Autodesk Fusion 360 part; units mm, degrees
sketch "Sketch1" plane through (0, 0, 0) normal (0, 1, 0) x (1, 0, 0)
sketch "Sketch2" plane through (0, 0, 0) normal (0, 1, 0) x (1, 0, 0)
sketch "Sketch3" plane through (0, 0, 0) normal (0, 1, 0) x (1, 0, 0)
  line L0 (-7.8, -52.8) -> (7.8, -52.8)
  line L1 (7.8, -52.8) -> (7.8, -37.2)
  line L2 (7.8, -37.2) -> (-7.8, -37.2)
  line L3 (-7.8, -37.2) -> (-7.8, -52.8)
  line L4 (-7.8, -52.8) -> (7.8, -37.2) construction
  line L5 (7.8, -52.8) -> (-7.8, -37.2) construction
  point P0 (0, -45)
  dimension "d3" = 15.6
  dimension "d4" = 15.6
extrude "Extrude1" add sketch "Sketch3" along normal blind 6.6 draft -20 makes body 1
sketch "Sketch4" plane through (0, 0, 0) normal (1, 0, 0) x (0, 0, -1)
extrude "Extrude2" add 1 faces at (-2.6, 0, 42.4) along direction (0, -1, 0) blind 5 draft -10 on bodies 1 bodies 1
sketch "Sketch5" plane through (0, 6.6, 0) normal (0, 1, 0) x (-1, 0, 0)
  line L0 (-5.3978, 39.6022) -> (5.3978, 39.6022)
  line L1 (5.3978, 39.6022) -> (5.3978, 50.3978)
  line L2 (5.3978, 50.3978) -> (-5.3978, 50.3978)
  line L3 (-5.3978, 50.3978) -> (-5.3978, 39.6022)
  line L4 (-3, 41) -> (3, 41)
  line L5 (3, 41) -> (3, 49)
  line L6 (3, 49) -> (-3, 49)
  line L7 (-3, 49) -> (-3, 41)
  line L8 (-3, 41) -> (3, 49) construction
  line L9 (3, 41) -> (-3, 49) construction
  point P0 (0, 45)
extrude "Extrude3" cut sketch "Sketch5" against normal blind 1 contours L4 L5 L6 L7 bodies 1
sketch "Sketch6" plane through (0, 5.6, 0) normal (0, 1, 0) x (-1, 0, 0)
  line L0 (-3, 49) -> (-3, 41)
  line L1 (-3, 41) -> (3, 41)
  line L2 (3, 41) -> (3, 49)
  line L3 (3, 49) -> (-3, 49)
  line L4 (2.8, 41.1) -> (-2.8305, 41.1)
  line L5 (-2.8305, 41.1) -> (-2.8305, 48.9)
  line L6 (-2.8305, 48.9) -> (2.8, 48.9)
  line L7 (2.8, 48.9) -> (2.8, 41.1)
  line L8 (2.8, 41.1) -> (-2.8305, 48.9) construction
  line L9 (-2.8305, 41.1) -> (2.8, 48.9) construction
  point P0 (-0.0152, 45)
extrude "Extrude4" add sketch "Sketch6" along normal blind 2 contours L4 L5 L6 L7 bodies 1
sketch "Sketch7" plane through (0, 7.6, 0) normal (0, 1, 0) x (-1, 0, 0)
  line L0 (2.8, 48.9) -> (-2.8305, 48.9)
  line L1 (-2.8305, 48.9) -> (-2.8305, 41.1)
  line L2 (-2.8305, 41.1) -> (2.8, 41.1)
  line L3 (2.8, 41.1) -> (2.8, 48.9)
  line L4 (0.6, 43.2) -> (-0.6, 43.2)
  line L5 (-0.6, 43.2) -> (-0.6, 46.8)
  line L6 (-0.6, 46.8) -> (0.6, 46.8)
  line L7 (0.6, 46.8) -> (0.6, 43.2)
  line L8 (0.6, 43.2) -> (-0.6, 46.8) construction
  line L9 (-0.6, 43.2) -> (0.6, 46.8) construction
  line L10 (-1.8, 44.4) -> (1.8, 44.4)
  line L11 (1.8, 44.4) -> (1.8, 45.6)
  line L12 (1.8, 45.6) -> (-1.8, 45.6)
  line L13 (-1.8, 45.6) -> (-1.8, 44.4)
  line L14 (-1.8, 44.4) -> (1.8, 45.6) construction
  line L15 (1.8, 44.4) -> (-1.8, 45.6) construction
  point P0 (0, 45)
  point P1 (0, 45)
extrude "Extrude5" add sketch "Sketch7" along normal blind 3.2 contours L4 L5 L7 L10 | L5 L7 L10 L12 | L7 L10 L11 L12 | L5 L10 L12 L13 | L5 L6 L7 L12 bodies 1
sketch "Sketch8" plane through (-2.8, 0, 0) normal (-1, 0, 0) x (0, 0, 1)
  line L0 (41.1, 5.6) -> (48.9, 5.6)
  line L1 (48.9, 5.6) -> (48.9, 7.6)
  line L2 (48.9, 7.6) -> (41.1, 7.6)
  line L3 (41.1, 7.6) -> (41.1, 5.6)
extrude "Extrude6" cut 1 faces at (1.4, 10.8, 45.2) along direction (0, -1, 0) blind 0.6 on bodies 1 bodies 1
sketch "Sketch9" plane through (0, -5, 0) normal (0, -1, 0) x (1, 0, 0)
  line L0 (6.9184, 51.9184) -> (-6.9184, 51.9184)
  line L1 (-6.9184, 51.9184) -> (-6.9184, 38.0816)
  line L2 (-6.9184, 38.0816) -> (6.9184, 38.0816)
  line L3 (6.9184, 38.0816) -> (6.9184, 51.9184)
  circle A0 centre (0, 45) radius 3
extrude "Extrude7" add sketch "Sketch9" along normal blind 2.5 contours A0 bodies 1
extrude "Extrude8" add 1 faces at (0.8808, -7.5, 44.8347) along direction (0, -1, 0) blind 0.8 draft -45 on bodies 1 bodies 1
sketch "Sketch10" plane through (0, -5, 0) normal (0, -1, 0) x (1, 0, 0)
  circle A0 centre (0, 45) radius 3
  line L0 (6.9184, 51.9184) -> (-6.9184, 51.9184)
  line L1 (-6.9184, 51.9184) -> (-6.9184, 38.0816)
  line L2 (-6.9184, 38.0816) -> (6.9184, 38.0816)
  line L3 (6.9184, 38.0816) -> (6.9184, 51.9184)
  circle A1 centre (-5, 42.5) radius 0.5
  circle A2 centre (5, 40) radius 0.5
extrude "Extrude9" add sketch "Sketch10" along normal blind 2.5 contours A1 | A2 bodies 1
extrude "Extrude10" add 2 faces at (-5.0609, -7.5, 42.6551) (4.9391, -7.5, 40.1551) along direction (0, -1, 0) blind 0.8 draft -25 on bodies 1 bodies 1
sketch "Sketch11" plane through (-2.8, 0, 0) normal (-1, 0, 0) x (0, 0, 1)
copy_body "Body->Comp1" bodies 1 removing the originals makes body 2 in component "Switch"
component "Switch" placed x (1, 0, 0) y (0, 1, 0) z (0, 0, 1) at (0, 0, 0)
Here's how the part is built. I have some questions about the finished solid (model axes, mm). A direction names the side the tool comes from. Round coordinates to 2 decimals unless told otherwise and drop trailing zeros. Write each loop counter-clockwise with the first axis right and the second up, starting at its lowest first coordinate (ties: lowest second). Pieces come first, ordered by that corner, then holes.
Q1. If we section it at A-A on z = 45: Write out the boundary of the cut face in (x, y).
Q2. If we section it at B-B on x = 0: Write out the boundary of the cut face in (y, z).
Q3. Please list where these lines run through material, in increasing order: probe 1 along Y at (x, z) = (1, 40.25); probe 2 along Z at (x, y) = (1.5, 8.75); probe 3 along Z at (x, y) = (-2, 7.25).
Q4. Which directions (+Z, -Z, +X, -X, +Y, -Y) give clear straight access to the entire face, cutting with the end or side of a thin tool? Please do faces 4 (the flat face through (-3, 6, 45)), 5 (the flat face through (0.6, 9, 46)), 6 (the flat face through (0.6, 9, 44)), 7 (the cylindrical face through (-5, -6, 43)), 8 (the flat face through (-1.8, 9, 45)).
Q5. If we section it at D-D on z = 41.5: Write out the boundary of the cut face in (x, y).
Q6. If we section it at C-C on y = -1.25: Write out the boundary of the cut face in (x, z), plus the area to 3 significant figures.
Q7. If we mould it in two halves opening along Z, with no side actions, what happens to faces 1 (the flat face through (-3.2, -5, 44.9)), 2 (the flat face through (-1, 9, 45.6)), 3 (the flat face through (0, 7, 48.9))? For each: +Z half, -Z half, draft (parallel to the pull), parting line (faces both ways), or undercut.
Q8. Will these pins go through, and if not, where does the flat tip stop? P1, Ø1, axis at x = -5, z = 39.5, coming from the +Y side; P2, Ø1.3, axis at x = 1.5, y = 8.5, coming from the +Z side; P3, Ø6, axis at x = -1.5, y = 0.5, coming from the +Z side.
Answer below:
1. outline: (-7.8, 0) - (-6.92, -5) - (-3, -5) - (-3, -7.5) - (-2.2, -8.3) - (2.2, -8.3) - (3, -7.5) - (3, -5) - (6.92, -5) - (7.8, 0) - (5.4, 6.6) - (3, 6.6) - (3, 5.6) - (2.83, 5.6) - (2.83, 7.6) - (1.8, 7.6) - (1.8, 10.2) - (-1.8, 10.2) - (-1.8, 7.6) - (-2.8, 7.6) - (-2.8, 5.6) - (-3, 5.6) - (-3, 6.6) - (-5.4, 6.6) - close
2. outline: (-8.3, 42.8) - (-7.5, 42) - (-5, 42) - (-5, 38.08) - (0, 37.2) - (6.6, 39.6) - (6.6, 41) - (5.6, 41) - (5.6, 41.1) - (7.6, 41.1) - (7.6, 43.2) - (10.2, 43.2) - (10.2, 46.8) - (7.6, 46.8) - (7.6, 48.9) - (5.6, 48.9) - (5.6, 49) - (6.6, 49) - (6.6, 50.4) - (0, 52.8) - (-5, 51.92) - (-5, 48) - (-7.5, 48) - (-8.3, 47.2) - close
3. probe 1: y = -5 to 6.6
3. probe 2: z = 44.4 to 45.6
3. probe 3: z = 41.1 to 48.9
4. face 4: +Y
4. face 5: +Z, +X, +Y
4. face 6: -Z, +X, +Y
4. face 7: -Y
4. face 8: +Z, -Z, -X, +Y
5. outline: (-7.8, 0) - (-6.92, -5) - (6.92, -5) - (7.8, 0) - (5.4, 6.6) - (3, 6.6) - (3, 5.6) - (2.83, 5.6) - (2.83, 7.6) - (-2.8, 7.6) - (-2.8, 5.6) - (-3, 5.6) - (-3, 6.6) - (-5.4, 6.6) - close
6. outline: (-7.58, 37.42) - (7.58, 37.42) - (7.58, 52.58) - (-7.58, 52.58) - close
6. area: 230 mm2
7. face 1: draft
7. face 2: +Z half
7. face 3: undercut
8. P1: stops at y = 6.6
8. P2: stops at z = 45.6
8. P3: stops at z = 52.8
